Design review of the part built by this model. Coordinates are the model's own, in mm. A direction names the side the tool comes from. Round coordinates to 2 decimals unless told otherwise and drop trailing zeros. Loops run counter-clockwise (first coordinate to the right, second up) from the corner with the lowest first, then second, coordinate; pieces in that order, holes last. Notation, with made-up numbers: (40.25, -27) - (48.25, -27) arc R31 cw to (48.25, 12) - close; hole circle Ø10 at (-36.5, 83.5). An arc over 180 degrees is marked (long way). Return JSON: item names as keys, results as strings. Group by question number.
from build123d import *

# Parameters (mm, degrees)
F0_W     = 22
F0_H     = 23
F1_DEPTH = 4.5
F2_R     = 1.75
F3_DEPTH = 4.501
F4_W     = 22
F4_H     = 6
F4_R     = 1.75
F5_DEPTH = 1.5
F2_W     = 22
F2_H     = 23
F2_R_2   = 4.25
F2_R_3   = 1.5
F6_DEPTH = 3
F7_R     = 1.5
F8_DEPTH = 3
F9_DEPTH = 9.001


with BuildPart() as f1:
    # F0 (on Top) → F1 (new body)
    with BuildSketch(Plane.XY):
        with Locations((1.9347620532, -2.93618536)):
            Rectangle(F0_W, F0_H)
    extrude(amount=F1_DEPTH)

    # F2 (on face) → F3 (cut, through all)
    with BuildSketch(Plane.XY.offset(4.5)):
        with Locations((1.9347620532, 1.31381464)):
            Circle(F2_R)
    extrude(amount=-F3_DEPTH, mode=Mode.SUBTRACT)

    # F4 (on face) → F5 (join)
    with BuildSketch(Plane(origin=(0, 0, 0), x_dir=(1, 0, 0), z_dir=(0, 0, -1))):
        with Locations((1.9347620532, -1.31381464)):
            Rectangle(F4_W, F4_H)
        with Locations((1.9347620532, -1.31381464)):
            Circle(F4_R, mode=Mode.SUBTRACT)
    extrude(amount=F5_DEPTH)

    # F2 (on face) → F6 (join)
    with BuildSketch(Plane.XY.offset(4.5)):
        with Locations((1.9347620532, -2.93618536)):
            Rectangle(F2_W, F2_H)
        Polygon((-5.8697039075, -7.3919604017), (-8.0607315208, -5.1739888063), (-7.235425581, -2.1675174351), (-4.2190920279, -1.3790176593), (-2.0280644146, -3.5969892546), (-2.8533703544, -6.6034606258), align=None, mode=Mode.SUBTRACT)
        with Locations((1.9347620532, 1.31381464)):
            Circle(F2_R_2, mode=Mode.SUBTRACT)
        Polygon((-7.235425581, -2.1675174351), (-8.0607315208, -5.1739888063), (-5.8697039075, -7.3919604017), (-2.8533703544, -6.6034606258), (-2.0280644146, -3.5969892546), (-4.2190920279, -1.3790176593), align=None)
        with Locations((-5.0443979677, -4.3854890305)):
            Circle(F2_R_3, mode=Mode.SUBTRACT)
        with Locations((-5.0443979677, -4.3854890305)):
            Circle(F2_R_3)
    extrude(amount=F6_DEPTH)

    # F7 (on face) → F8 (cut)
    with BuildSketch(Plane.XY.offset(7.5)):
        Polygon((-2.0280644146, -3.5969892546), (-4.2190920279, -1.3790176593), (-7.235425581, -2.1675174351), (-8.0607315208, -5.1739888063), (-5.8697039075, -7.3919604017), (-2.8533703544, -6.6034606258), align=None)
        with Locations((-5.0443979677, -4.3854890305)):
            Circle(F7_R, mode=Mode.SUBTRACT)
    extrude(amount=-F8_DEPTH, mode=Mode.SUBTRACT)

    # F9 (cut, through all): a face of the model
    f9_faces = [f1.faces().sort_by_distance(p)[0] for p in [
        (-5.0443979677, -4.3854890305, 7.5),
    ]]
    extrude(f9_faces, amount=-F9_DEPTH, mode=Mode.SUBTRACT)


solid = f1.part
Q1. Draft analysis for pull direction Y (two halves, no side actions). For faces 4 (the flat face through (2, -1, -1.5)), 5 (the cylindrical face through (-5.37, -5.85, 2.28)), 6 (the flat face through (2, 4.314, -1)), state which applies: pulls with the +Y half, pulls with the -Y half, needs draft (parallel to the pull), parting line crosses it, or undercut.
Q2. Add section D-D, the plane z = -0.5. State the section outline as (x, y) points, plus the area to 3 significant figures.
Q3. Add section B-B, the plane y = -4. State the section outline as (x, z) points, plus the area to 3 significant figures.
Q4. Add section A-A, the plane x = 2.25. State the section outline as (y, z) points.
Q5. Tool access review of faces 1 (the flat face through (-7.642, -3.65, 6.021)), 2 (the flat face through (2, 6, 0)), 3 (the flat face through (2, 8.564, 4)): name each direction out of +Z, -Z, +X, -X, +Y, -Y from which nothing blocks a thin tool from reaching the whole face with its end or side.
Q6. Insertion check: pin 1 Ø10 at (x, y) = (1.93, 1.31) entering from -Z; pin 2 Ø5 at (x, y) = (10.5, -12) entering from -Z; pin 3 Ø4 at (x, y) = (1.93, 1.31) entering from +Z; pin 4 Ø0.8 at (x, z) = (0, -0.5) entering from -Y. Each pin has a flat end and moves straight along its axis. Give the tip position at first contact, or say it passes through.
Q7. Add section C-C, the plane x = 10.75. State the section outline as (y, z) points.
Q8. For line 1 (Z direction, x = -0.25, y = -5); line 2 (X direction, y = 2, z = 6); line 3 (Y direction, x = 7, z = -0.5), list the stretches that pass through material, from the lowest coordinate up.
Evaluation:
{
 "1": {"face 4": "needs draft", "face 5": "undercut", "face 6": "pulls with the +Y half"},
 "2": {"outline": "(-9.07, -1.69) - (12.93, -1.69) - (12.93, 4.31) - (-9.07, 4.31) - close; hole circle Ø3.5 at (1.93, 1.31)", "area": "122 mm²"},
 "3": {"outline": "(-9.07, 0) - (-6.49, 0) - (-6.49, 4.5) - (-7.74, 4.5) - (-7.74, 7.5) - (-9.07, 7.5) - close; (-3.59, 0) - (12.93, 0) - (12.93, 7.5) - (-2.14, 7.5) - (-2.14, 4.5) - (-3.59, 4.5) - close", "area": "135 mm²"},
 "4": {"outline": "(-14.44, 0) - (-1.69, 0) - (-1.69, -1.5) - (-0.41, -1.5) - (-0.41, 4.5) - (-2.92, 4.5) - (-2.92, 7.5) - (-14.44, 7.5) - close; (3.04, -1.5) - (4.31, -1.5) - (4.31, 0) - (8.56, 0) - (8.56, 7.5) - (5.55, 7.5) - (5.55, 4.5) - (3.04, 4.5) - close"},
 "5": {"face 1": "+Z", "face 2": "-Z, +X, -X, +Y", "face 3": "+Z, -Z, +X, -X, +Y"},
 "6": {"pin 1": "z = -1.5", "pin 2": "z = 0", "pin 3": "z = 4.5", "pin 4": "y = -1.69"},
 "7": {"outline": "(-14.44, 0) - (-1.69, 0) - (-1.69, -1.5) - (4.31, -1.5) - (4.31, 0) - (8.56, 0) - (8.56, 7.5) - (-14.44, 7.5) - close"},
 "8": {"line 1": "0 to 7.5", "line 2": "-9.07 to -2.26, 6.13 to 12.93", "line 3": "-1.69 to 4.31"}
}
